Source: CAD feature listing. Evaluate the final solid. Frame: model axes, mm. Face numbers are marked on the shaded views. A direction names the side the tool comes from. Coordinates: 2 decimals unless noted, no trailing zeros. Order: outer loops, then holes, each group sorted by start corner. A loop starts at its lowest first (then second) coordinate and runs counter-clockwise, first axis right, second up.
```python
from build123d import *

# Parameters (mm, degrees)
SKETCH1_W                = 80
SKETCH1_H                = 52
BOSS_EXTRUDE1_DEPTH      = 2
SKETCH2_W                = 93.1
SKETCH2_H                = 9.8
BOSS_EXTRUDE2_DEPTH      = 3.3
BOSS_EXTRUDE3_DEPTH      = 13
BOSS_EXTRUDE3_DEPTH_BACK = 2
SKETCH3_W                = 97.1
SKETCH3_H                = 95.1
SKETCH3_W_2              = 93.1
SKETCH3_H_2              = 91.1
SKETCH4_R                = 3.5
CUT_EXTRUDE1_DEPTH       = 29
SKETCH5_R                = 2.5
CUT_EXTRUDE2_DEPTH       = 29


with BuildPart() as part:
    # Sketch1 → Boss-Extrude1 (new body)
    with BuildSketch(Plane.XY):
        Polygon((-46.55, -35.4), (-46.55, -55.7), (46.55, -55.7), (46.55, -35.4), (46.55, 35.4), (-46.55, 35.4), align=None)
        Rectangle(SKETCH1_W, SKETCH1_H, mode=Mode.SUBTRACT)
    extrude(amount=BOSS_EXTRUDE1_DEPTH)

    # Sketch2 → Boss-Extrude2 (add)
    with BuildSketch(Plane(origin=(0, 0, 0), x_dir=(-1, 0, 0), z_dir=(0, 0, -1))):
        with Locations((0, -30.9)):
            Rectangle(SKETCH2_W, SKETCH2_H)
    extrude(amount=BOSS_EXTRUDE2_DEPTH)

    # Sketch3 → Boss-Extrude3 (add, two sides: drawn at the far end of the back side and taken through both)
    with BuildSketch(Plane(origin=(0, 0, 0), x_dir=(-1, 0, 0), z_dir=(0, 0, -1)).offset(-BOSS_EXTRUDE3_DEPTH_BACK)):
        with Locations((0, -10.15)):
            Rectangle(SKETCH3_W, SKETCH3_H)
        with Locations((0, -10.15)):
            Rectangle(SKETCH3_W_2, SKETCH3_H_2, mode=Mode.SUBTRACT)
    extrude(amount=BOSS_EXTRUDE3_DEPTH + BOSS_EXTRUDE3_DEPTH_BACK)

    # Sketch4 → Cut-Extrude1 (cut)
    with BuildSketch(Plane.XY.offset(2)):
        with Locations((17.55, -45.4)):
            Circle(SKETCH4_R)
    extrude(amount=-CUT_EXTRUDE1_DEPTH, mode=Mode.SUBTRACT)

    # Sketch5 → Cut-Extrude2 (cut)
    with BuildSketch(Plane.XY.offset(2)):
        with Locations((2.55, -47.4)):
            Circle(SKETCH5_R)
        with Locations((34.95, -47.4)):
            Circle(SKETCH5_R)
    extrude(amount=-CUT_EXTRUDE2_DEPTH, mode=Mode.SUBTRACT)


solid = part.part
```
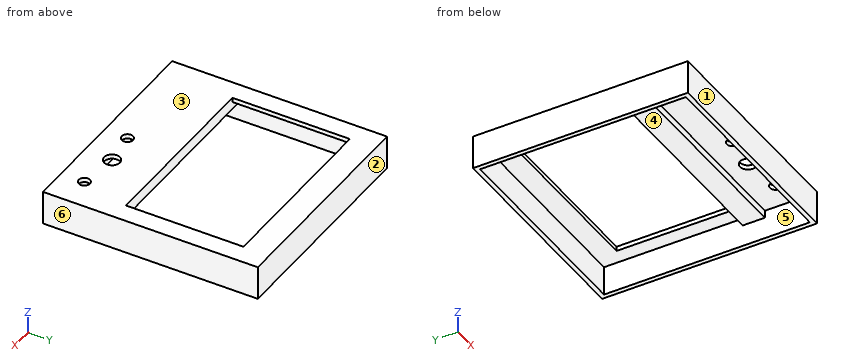
1. Section query D-D, the plane y = -47.4. Output: boundary loops of the cut face in (x, z).
2. Material intervals for line 1 along Y through (x, z) = (17.55, 0.75); line 2 along Y through (x, z) = (34.95, 1.4); line 3 along Y through (x, z) = (6.5, 1), sorted ascending.
3. Section query A-A, the plane x = 34.95. Output: boundary loops of the cut face in (y, z), plus the area to 3 significant figures.
4. Section query B-B, the plane y = -13. Output: boundary loops of the cut face in (x, z), plus the area to 3 significant figures.
5. Contact query for flat-ended pins moving along their axis: P1, Ø6, axis at x = 2.55, y = -47.4, coming from the +Z side; P2, Ø11, axis at x = 17.5, y = -29, coming from the -Z side; P3, Ø6, axis at x = -15.5, y = -49, coming from the -Z side. Output: stop coordinate, or through.
6. Section query C-C, the plane z = -2. Output: boundary loops of the cut face in (x, y), plus the area to 3 significant figures.
7. Draft query along Y for the marked faces 1, 2, 3 and 4. Return one class per face: +Y half, -Y half, draft (parallel to the pull), parting line (faces both ways), or undercut.
8. Access query for the marked faces 5 and 6. Directions: +Z, -Z, +X, -X, +Y, -Y. A direction counts if a zero-diameter tool reaches every point of the face in a straight line with its end or side. Return the directions, or none.
Answer key:
1. outline: (-48.55, -13) - (-46.55, -13) - (-46.55, 0) - (0.05, 0) - (0.05, 2) - (-48.55, 2) - close; (5.05, 0) - (14.68, 0) - (14.68, 2) - (5.05, 2) - close; (20.42, 0) - (32.45, 0) - (32.45, 2) - (20.42, 2) - close; (37.45, 0) - (46.55, 0) - (46.55, -13) - (48.55, -13) - (48.55, 2) - (37.45, 2) - close
2. line 1: y = -57.7 to -48.9, -41.9 to -26, 26 to 37.4
2. line 2: y = -57.7 to -49.9, -44.9 to -26, 26 to 37.4
2. line 3: y = -57.7 to -26, 26 to 37.4
3. outline: (-57.7, -13) - (-55.7, -13) - (-55.7, 0) - (-49.9, 0) - (-49.9, 2) - (-57.7, 2) - close; (-44.9, 0) - (-35.8, 0) - (-35.8, -3.3) - (-26, -3.3) - (-26, 2) - (-44.9, 2) - close; (26, 0) - (35.4, 0) - (35.4, -13) - (37.4, -13) - (37.4, 2) - (26, 2) - close
3. area: 161 mm2
4. outline: (-48.55, -13) - (-46.55, -13) - (-46.55, 0) - (-40, 0) - (-40, 2) - (-48.55, 2) - close; (40, 0) - (46.55, 0) - (46.55, -13) - (48.55, -13) - (48.55, 2) - (40, 2) - close
4. area: 86.2 mm2
5. P1: stops at z = 2
5. P2: stops at z = -3.3
5. P3: stops at z = 0
6. outline: (-48.55, -57.7) - (48.55, -57.7) - (48.55, 37.4) - (-48.55, 37.4) - close; hole (-46.55, -55.7) - (46.55, -55.7) - (46.55, -35.8) - (-46.55, -35.8) - close; hole (-46.55, -26) - (46.55, -26) - (46.55, 35.4) - (-46.55, 35.4) - close
6. area: 1,670 mm2
7. face 1: -Y half
7. face 2: +Y half
7. face 3: draft
7. face 4: undercut
8. face 5: -Z
8. face 6: +Z, -Z, +X, +Y, -Y
